Check sheet for the drawn part. Datum: minimum x, y, z corner. Units: mm. Coordinates: 2 decimals unless noted, no trailing zeros. Write each loop counter-clockwise with the first axis right and the second up, starting at its lowest first coordinate (ties: lowest second). Pieces come first, ordered by that corner, then holes. Notation, with made-up numbers: M 70.5,53.5 L 129.5,53.5 A17 ccw 129.5,69.5 Z; hole C -18,60 d7. An arc over 180 degrees is marked long. Answer as a JSON object with one key per item and string values. Group by question number.
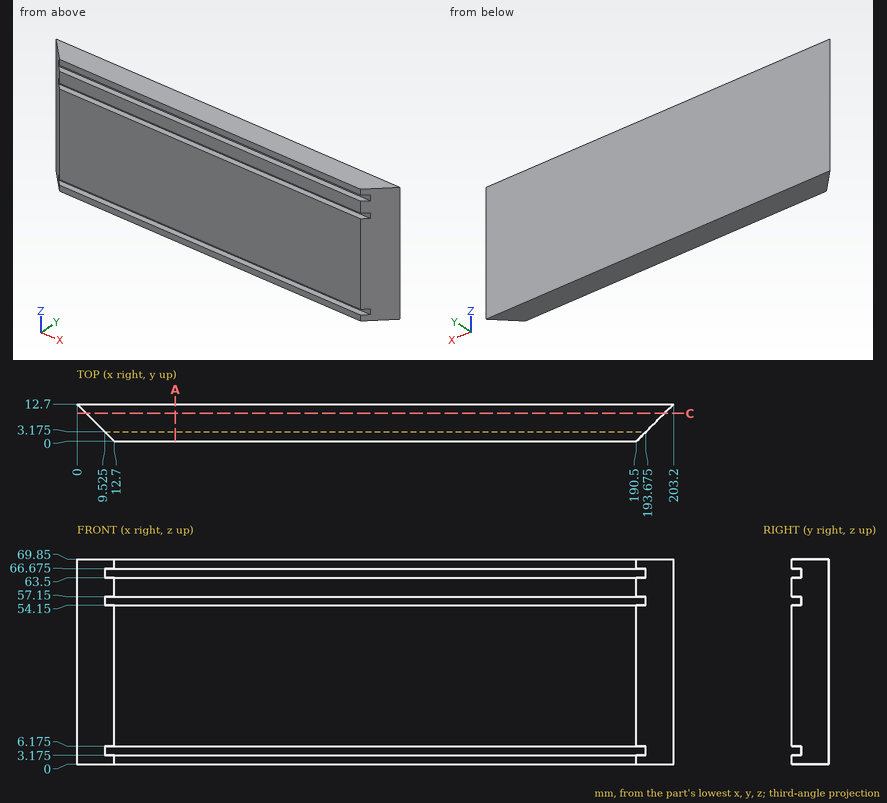
1) Section check C-C (y = 9.5). Record the cut outline in (x, z), then the cut area to 3 significant figures.
2) Material ranges on probe 1 along Z at (x, y) = (154.5, 2.25) (3 decimals); probe 2 along Y at (x, z) = (92, 5) (3 decimals); probe 3 along X at (y, z) = (2.25, 16), recorded low to high. Write a range as [from, to].
3) Section check A-A (x = 33.5). Record the cut outline in (y, z) (3 decimals), then the cut area to 3 significant figures.
4) Go/stop test with flat-tipped pins: pin 1 Ø1.5 at (x, z) = (141.5, 4) entering from -Y (3 decimals); pin 2 Ø3 at (y, z) = (9, 40.5) entering from -X; pin 3 Ø1.5 at (y, z) = (4.5, 53) entering from +X. Record where each tip stops, or that it passes through.
Entries:
{
 "1": {"outline": "M 3.2,0 L 200,0 L 200,69.85 L 3.2,69.85 Z", "area": "13,700 mm^2"},
 "2": {"probe 1": "[0, 3.175], [6.175, 54.15], [57.15, 63.5], [66.675, 69.85]", "probe 2": "[3.175, 12.7]", "probe 3": "[10.45, 192.75]"},
 "3": {"outline": "M 0,0 L 12.7,0 L 12.7,69.85 L 0,69.85 L 0,66.675 L 3.175,66.675 L 3.175,63.5 L 0,63.5 L 0,57.15 L 3.175,57.15 L 3.175,54.15 L 0,54.15 L 0,6.175 L 3.175,6.175 L 3.175,3.175 L 0,3.175 Z", "area": "858 mm^2"},
 "4": {"pin 1": "y = 3.175", "pin 2": "x = 2.2", "pin 3": "x = 195.75"}
}
